Can you work these out from the model? Positions are in its coordinate system, mm. A direction names the side the tool comes from. Round coordinates to 2 decimals unless told otherwise and drop trailing zeros. Order: outer loops, then holes, each group sorted by start corner. A loop starts at its lowest first (then second) coordinate and runs counter-clockwise, first axis right, second up. Notation, with made-up numbers: M -15.5,-26 L -2.5,-26 A20 cw -2.5,3 Z; hole C -23.75,47 d9. An arc over 180 degrees is marked long. Answer as a JSON object with one key per item and string values. Group by question number.
```python
from build123d import *

# Parameters (mm, degrees)
SKETCH2_R           = 3.06197
BOSS_EXTRUDE1_DEPTH = 31.75
SKETCH3_R           = 8.382
BOSS_EXTRUDE2_DEPTH = 16.9164
SKETCH4_R           = 2.9972
CUT_EXTRUDE1_DEPTH  = 13.97
SKETCH5_R           = 2.2225
CUT_EXTRUDE2_DEPTH  = 13.97


with BuildPart() as part:
    # Sketch2 → Boss-Extrude1 (new body)
    with BuildSketch(Plane.XY):
        Circle(SKETCH2_R)
    extrude(amount=BOSS_EXTRUDE1_DEPTH)

    # Sketch3 → Boss-Extrude2 (add)
    with BuildSketch(Plane(origin=(0, 0, 0), x_dir=(-1, 0, 0), z_dir=(0, 0, -1))):
        Circle(SKETCH3_R)
    extrude(amount=BOSS_EXTRUDE2_DEPTH)

    # Sketch4 → Cut-Extrude1 (cut)
    with BuildSketch(Plane(origin=(0, 0, -16.9164), x_dir=(-1, 0, 0), z_dir=(0, 0, -1))):
        Circle(SKETCH4_R)
    extrude(amount=-CUT_EXTRUDE1_DEPTH, mode=Mode.SUBTRACT)

    # Sketch5 → Cut-Extrude2 (cut)
    with BuildSketch(Plane(origin=(0, 0, 0), x_dir=(1, 0, 0), z_dir=(0, 1, 0))):
        with Locations((0, 8.4582)):
            Circle(SKETCH5_R)
    extrude(amount=CUT_EXTRUDE2_DEPTH, mode=Mode.SUBTRACT)


solid = part.part
```
1) If we section it at D-D on y = 5.5: Write out the boundary of the cut face in (x, z) (1 decimal), plus the area to 3 significant figures.
2) If we section it at B-B on y = 0: Write out the boundary of the cut face in (x, z).
3) We'd pull the mould along X, two halves only. Please class faces 1 (the face through (0, 0, 31.75)), 2 (the face through (1.82, -8.18, -8.34)), 3 (the face through (2.053, 5.156, -7.607)): +X half, -X half, draft (parallel to the pull), parting line (faces both ways), or undercut.
4) For pin 1 (3.5 mm diameter, centred on x = 0, y = 0, fed in from -Z); pin 2 (1 mm diameter, centred on x = 1.5, z = 16.5, fed in from +Y); pin 3 (2 mm diameter, centred on x = -4.5, y = 5, fed in from +Z), each with a flat end and sliding along its axis, tell me the tip position at first contact or that it passes through.
5) Which directions (+Z, -Z, +X, -X, +Y, -Y) give clear straight access to the entire face, cutting with the end or side of a thin tool? Please do faces 4 (the face through (0, 0, -2.946)), 5 (the face through (0, -4, -16.916)), 6 (the face through (-3.06, 0.13, 15.65)).
6) If we section it at A-A on x = 0: Write out the boundary of the cut face in (y, z).
7) If we section it at C-C on z = -14: Write out the boundary of the cut face in (x, y).
8) I need wall thicknesses on line 1 along Z through (x, y) = (0, 7); line 2 along Y through (x, z) = (0, -12.75); line 3 along Z through (x, y) = (2.5, -2.5). Which ranges of each line are inside material? Lowest first, please.
Findings:
{
 "1": {"outline": "M -6.3,-16.9 L 6.3,-16.9 L 6.3,0 L -6.3,0 Z; hole C 0,-8.5 d4.4", "area": "198 mm^2"},
 "2": {"outline": "M -8.38,-16.92 L -3,-16.92 L -3,-2.95 L 3,-2.95 L 3,-16.92 L 8.38,-16.92 L 8.38,0 L 3.06,0 L 3.06,31.75 L -3.06,31.75 L -3.06,0 L -8.38,0 Z"},
 "3": {"face 1": "draft", "face 2": "parting line", "face 3": "undercut"},
 "4": {"pin 1": "stops at z = -2.95", "pin 2": "stops at y = 2.89", "pin 3": "stops at z = 0"},
 "5": {"face 4": "-Z", "face 5": "-Z, +X, -X, +Y, -Y", "face 6": "+Z"},
 "6": {"outline": "M -8.38,-16.92 L -3,-16.92 L -3,-2.95 L 3,-2.95 L 3,-6.24 L 8.38,-6.24 L 8.38,0 L 3.06,0 L 3.06,31.75 L -3.06,31.75 L -3.06,0 L -8.38,0 Z; M 3,-16.92 L 8.38,-16.92 L 8.38,-10.68 L 3,-10.68 Z"},
 "7": {"outline": "C 0,0 d16.76; hole C 0,0 d5.99"},
 "8": {"line 1": "z = -16.92 to -10.68, -6.24 to 0", "line 2": "y = -8.38 to -3, 3 to 8.38", "line 3": "z = -16.92 to 0"}
}
